```python
from build123d import *

# Parameters (mm, degrees)
F0_R     = 1.5
F1_DEPTH = 10


with BuildPart() as f1:
    # F0 (on Front) → F1 (new body)
    with BuildSketch(Plane.XZ):
        with BuildLine():
            Line((-15, -20), (15, -20))
            ThreePointArc((15, -20), (18.535534, -18.535534), (20, -15))
            Line((20, -15), (20, 15))
            ThreePointArc((20, 15), (18.535534, 18.535534), (15, 20))
            Line((15, 20), (-15, 20))
            ThreePointArc((-15, 20), (-18.535534, 18.535534), (-20, 15))
            Line((-20, 15), (-20, -15))
            ThreePointArc((-20, -15), (-18.535534, -18.535534), (-15, -20))
        make_face()
        with Locations((-16, -16)):
            Circle(F0_R, mode=Mode.SUBTRACT)
        with Locations((16, -16)):
            Circle(F0_R, mode=Mode.SUBTRACT)
        with Locations((-16, 16)):
            Circle(F0_R, mode=Mode.SUBTRACT)
        with BuildLine():
            ThreePointArc((1.5, 18.940697), (13.955286, 12.893797), (19, 0))
            ThreePointArc((19, 0), (18.53253, -4.188713), (17.153125, -8.17131))
            ThreePointArc((17.153125, -8.17131), (16.454483, -9.5), (15.653125, -10.769387))
            ThreePointArc((15.653125, -10.769387), (0, -19), (-15.653125, -10.769387))
            ThreePointArc((-15.653125, -10.769387), (-16.454483, -9.5), (-17.153125, -8.17131))
            ThreePointArc((-17.153125, -8.17131), (-16.454483, 9.5), (-1.5, 18.940697))
            ThreePointArc((-1.5, 18.940697), (0, 19), (1.5, 18.940697))
        make_face(mode=Mode.SUBTRACT)
        with Locations((16, 16)):
            Circle(F0_R, mode=Mode.SUBTRACT)
        with BuildLine():
            Line((1.5, 9.88686), (1.5, 18.940697))
            ThreePointArc((1.5, 18.940697), (0, 19), (-1.5, 18.940697))
            Line((-1.5, 18.940697), (-1.5, 9.88686))
            ThreePointArc((-1.5, 9.88686), (0, 10), (1.5, 9.88686))
        make_face()
        with BuildLine():
            Line((-9.312272, -3.644392), (-17.153125, -8.17131))
            ThreePointArc((-17.153125, -8.17131), (-16.454483, -9.5), (-15.653125, -10.769387))
            Line((-15.653125, -10.769387), (-7.812272, -6.242468))
            ThreePointArc((-7.812272, -6.242468), (-8.660254, -5), (-9.312272, -3.644392))
        make_face()
        with BuildLine():
            ThreePointArc((15.653125, -10.769387), (16.454483, -9.5), (17.153125, -8.17131))
            Line((17.153125, -8.17131), (9.312272, -3.644392))
            ThreePointArc((9.312272, -3.644392), (8.660254, -5), (7.812272, -6.242468))
            Line((7.812272, -6.242468), (15.653125, -10.769387))
        make_face()
        with BuildLine():
            ThreePointArc((10, 0), (7.582875, 6.519202), (1.5, 9.88686))
            ThreePointArc((1.5, 9.88686), (0, 10), (-1.5, 9.88686))
            ThreePointArc((-1.5, 9.88686), (-8.660254, 5), (-9.312272, -3.644392))
            ThreePointArc((-9.312272, -3.644392), (-8.660254, -5), (-7.812272, -6.242468))
            ThreePointArc((-7.812272, -6.242468), (0, -10), (7.812272, -6.242468))
            ThreePointArc((7.812272, -6.242468), (8.660254, -5), (9.312272, -3.644392))
            ThreePointArc((9.312272, -3.644392), (9.826564, -1.854357), (10, 0))
        make_face()
    extrude(amount=F1_DEPTH)


solid = f1.part
```
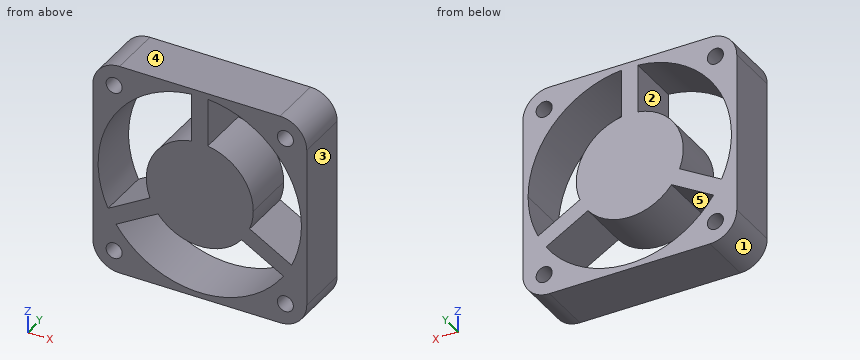
Work out the finished part from the listing and answer in its coordinate system (mm). Face numbers are marked on the shaded views. A direction names the side the tool comes from. Give positions to 0.01 mm unless a question says otherwise; leave off trailing zeros. Loops run counter-clockwise (first coordinate to the right, second up) from the corner with the lowest first, then second, coordinate; pieces in that order, holes last. Notation, with made-up numbers: (89, 68.25) -> (108, 68.25) arc R18 cw to (108, 72.25) -> close; hole circle Ø8 at (55, 17). An arc over 180 degrees is marked (long way). Put each result on its own line as item: value. Start each with the question number.
Item 1: The mould has two halves that part along X. Classify the marked faces 1, 2 and 3: released by +X, released by -X, zero draft, split by the parting line, or undercut.
Item 2: Each of these flat-tipped pins is pushed along its axis until it touches: P1, Ø1.8, axis at x = 16, z = 16, coming from the -Y side; P2, Ø2.5, axis at y = -3, z = 16.5, coming from the +X side. Where does it stop, or does it pass through?
Item 3: Find the intervals of material crossed by L1, parallel to Z at x = 2.5, y = -0.75; L2, parallel to Z at x = -12, y = -0.75; L3, parallel to X at y = -8.5, z = 5, in increasing order. Write a range as [from, to].
Item 4: The part is cut by section C-C (z = 16). Give the vertices of the cut face in (x, y).
Item 5: The part is cut by section D-D (z = 5). Give the vertices of the cut face in (x, y).
Item 6: Which of the six approach directions +Z, -Z, +X, -X, +Y, -Y give full straight-line access (tool end or side, diameter ignored) to the marked faces 4 and 5?
Item 7: The part is cut by section A-A (y = -1). Give the vertices of the cut face in (x, z), then the cut area to 3 significant figures.
Item 8: The part is cut by section B-B (x = -13). Give the vertices of the cut face in (y, z), then the cut area to 3 significant figures.
Answers below:
1. face 1: released by -X
1. face 2: undercut
1. face 3: released by +X
2. P1: through
2. P2: x = 19.99
3. L1: [-20, -18.83], [-9.68, 9.68], [18.83, 20]
3. L2: [-20, -14.73], [-8.66, -5.2], [14.73, 20]
3. L3: [-20, -18.33], [-8.66, 8.66], [18.33, 20]
4. outline: (-19.9, -10) -> (-17.5, -10) -> (-17.5, 0) -> (-19.9, 0) -> close; (-14.5, -10) -> (-10.25, -10) -> (-10.25, 0) -> (-14.5, 0) -> close; (-1.5, -10) -> (1.5, -10) -> (1.5, 0) -> (-1.5, 0) -> close; (10.25, -10) -> (14.5, -10) -> (14.5, 0) -> (10.25, 0) -> close; (17.5, -10) -> (19.9, -10) -> (19.9, 0) -> (17.5, 0) -> close
5. outline: (-20, -10) -> (-18.33, -10) -> (-18.33, 0) -> (-20, 0) -> close; (-8.66, -10) -> (8.66, -10) -> (8.66, 0) -> (-8.66, 0) -> close; (18.33, -10) -> (20, -10) -> (20, 0) -> (18.33, 0) -> close
6. face 4: +Z, +X, -X, +Y, -Y
6. face 5: +Y, -Y
7. outline: (-20, -15) arc R5 ccw to (-15, -20) -> (15, -20) arc R5 ccw to (20, -15) -> (20, 15) arc R5 ccw to (15, 20) -> (-15, 20) arc R5 ccw to (-20, 15) -> close; hole circle Ø3 at (-16, -16); hole circle Ø3 at (-16, 16); hole (-17.15, -8.17) -> (-9.31, -3.64) arc R10 cw to (-1.5, 9.89) -> (-1.5, 18.94) arc R19 ccw to start; hole (-15.65, -10.77) arc R19 ccw to (15.65, -10.77) -> (7.81, -6.24) arc R10 cw to (-7.81, -6.24) -> close; hole (1.5, 9.89) arc R10 cw to (10, 0) arc R10 cw to (9.31, -3.64) -> (17.15, -8.17) arc R19 ccw to (19, 0) arc R19 ccw to (1.5, 18.94) -> close; hole circle Ø3 at (16, -16); hole circle Ø3 at (16, 16)
7. area: 811 mm2
8. outline: (-10, -20) -> (0, -20) -> (0, -13.86) -> (-10, -13.86) -> close; (-10, -9.24) -> (0, -9.24) -> (0, -5.77) -> (-10, -5.77) -> close; (-10, 13.86) -> (0, 13.86) -> (0, 20) -> (-10, 20) -> close
8. area: 158 mm2
